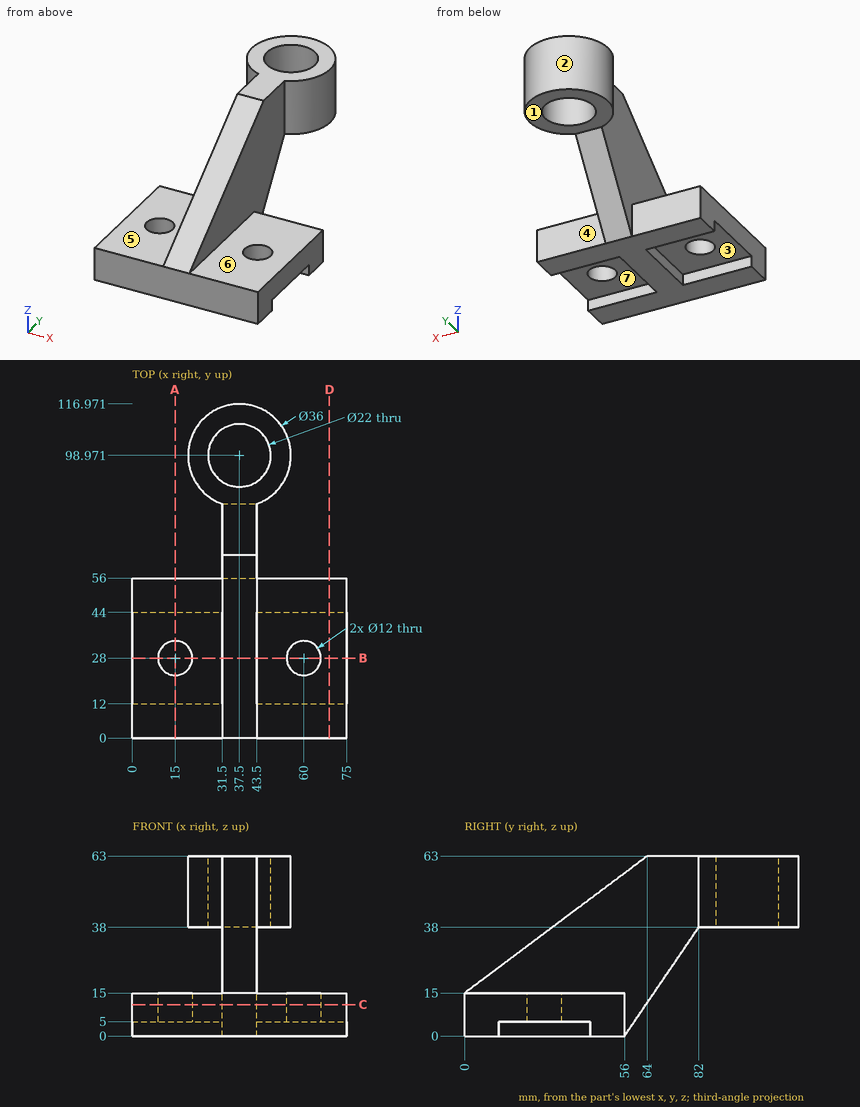
The drawing under review shows one solid part. Ordinate dimensions are in mm from its lowest x, y, z. A direction names the side the tool comes from. Coordinates: 2 decimals unless noted, no trailing zeros. Loops run counter-clockwise (first coordinate to the right, second up) from the corner with the lowest first, then second, coordinate; pieces in that order, holes last. Notation, with made-up numbers: (60.5, 27) - (106.5, 27) arc R4 ccw to (106.5, 34) - close; hole circle Ø5 at (-36, 88.5). An arc over 180 degrees is marked (long way). Use CSV: the item, a comma, the result in double quotes. Start each with the question number.
1. Add section D-D on x = 69. Give the boundary of the cut face in (y, z).
2. To check wall thickness, follow probe 1 along Y at (x, z) = (60, 7); probe 2 along Z at (x, y) = (49.5, 35.5); probe 3 along X at (y, z) = (18, 23). State the ranges of each line that lie inside material, in increasing order.
3. Clearance check with flat-ended pins moving along their axes: pin 1 (1.5 mm diameter, centred on x = 42.5, z = 23.5, fed in from +Y); pin 2 (1 mm diameter, centred on y = 96.5, z = 51, fed in from -X); pin 3 (8 mm diameter, centred on y = 36, z = 45.5, fed in from -X); pin 4 (20 mm diameter, centred on x = 37.5, y = 98.97, fed in from +Z). State where each tip first meets the part, or that it passes through.
4. Mouldability with a two-part tool opening along Y and no side actions: class the marked faces 1, 2 and 3 as released by +Y, released by -Y, zero draft, split by the parting line, or undercut.
5. Add section C-C on z = 11. Give the boundary of the cut face in (x, y).
6. Add section A-A on x = 15. Give the boundary of the cut face in (y, z), plus the area to 3 significant figures.
7. For the marked faces 4, 5, 6 and 7, list the 3-axis set-ups (+Z, -Z, +X, -X, +Y, -Y) from which the entire face can be reached by the end or side of a thin tool; tool diameter is ignored.
8. Add section B-B on y = 28. Give the boundary of the cut face in (x, z).
Resolved:
1,outline,"(0, 0) - (12, 0) - (12, 5) - (44, 5) - (44, 0) - (56, 0) - (56, 15) - (0, 15) - close"
2,probe 1,"0 to 22, 34 to 56"
2,probe 2,"5 to 15"
2,probe 3,"31.5 to 43.5"
3,pin 1,"y = 72.59"
3,pin 2,"x = 19.61"
3,pin 3,"x = 31.5"
3,pin 4,"through"
4,face 1,"zero draft"
4,face 2,"split by the parting line"
4,face 3,"undercut"
5,outline,"(0, 0) - (75, 0) - (75, 56) - (43.5, 56) - (43.5, 63.53) - (31.5, 63.53) - (31.5, 56) - (0, 56) - close; hole circle Ø12 at (15, 28); hole circle Ø12 at (60, 28)"
6,outline,"(0, 0) - (12, 0) - (12, 5) - (22, 5) - (22, 15) - (0, 15) - close; (34, 5) - (44, 5) - (44, 0) - (56, 0) - (56, 15) - (34, 15) - close"
6,area,"560 mm2"
7,face 4,"+Z, -Z, +X, +Y"
7,face 5,"+Z, -X, +Y, -Y"
7,face 6,"+Z, +X, +Y, -Y"
7,face 7,"-Z, +X"
8,outline,"(0, 5) - (9, 5) - (9, 15) - (0, 15) - close; (21, 5) - (31.5, 5) - (31.5, 0) - (43.5, 0) - (43.5, 5) - (54, 5) - (54, 15) - (43.5, 15) - (43.5, 36) - (31.5, 36) - (31.5, 15) - (21, 15) - close; (66, 5) - (75, 5) - (75, 15) - (66, 15) - close"
